Check sheet for the modelled part. Datum: model origin and axes. Units: mm. A direction names the side the tool comes from. Round coordinates to 2 decimals unless told otherwise and drop trailing zeros. Write each loop counter-clockwise with the first axis right and the second up, starting at its lowest first coordinate (ties: lowest second). Pieces come first, ordered by that corner, then holes. Notation, with made-up numbers: (82.25, -34) -> (118.25, -34) arc R15 cw to (118.25, -24) -> close; hole circle Ø1 at (8.5, 70.5). An arc over 180 degrees is marked (long way). One line per item, written item: value.
from build123d import *

# Parameters (mm, degrees)
SKETCH2_R          = 6.746875
CUT_EXTRUDE1_DEPTH = 12.1252


with BuildPart() as part:
    # Sketch1 → Revolve1 (revolve)
    with BuildSketch(Plane.XY):
        with BuildLine():
            Line((0, 0), (0, 11.1252))
            Line((0, 11.1252), (19.05, 11.1252))
            Line((19.05, 11.1252), (19.05, 4.7752))
            Line((19.05, 4.7752), (25.4, 4.7752))
            Line((25.4, 4.7752), (25.4, 0.79375))
            ThreePointArc((25.4, 0.79375), (25.167516008, 0.232483992), (24.60625, 0))
            Line((24.60625, 0), (0, 0))
        make_face()
    revolve(axis=Axis((0, 140.214345547, 0), (0, -1, 0)))

    # Sketch2 → Cut-Extrude1 (cut, through all)
    with BuildSketch(Plane(origin=(0, 11.1252, 0), x_dir=(1, 0, 0), z_dir=(0, 1, 0))):
        Circle(SKETCH2_R)
    extrude(amount=-CUT_EXTRUDE1_DEPTH, mode=Mode.SUBTRACT)


solid = part.part
Item 1: Sectioned sample at B-B on z = 0. Enter the section's corners in (x, y), and give its area (3 significant figures).
Answer:
outline: (-25.4, 0.79) arc R0.79 ccw to (-24.61, 0) -> (-6.75, 0) -> (-6.75, 11.13) -> (-19.05, 11.13) -> (-19.05, 4.78) -> (-25.4, 4.78) -> close; (6.75, 0) -> (24.61, 0) arc R0.79 ccw to (25.4, 0.79) -> (25.4, 4.78) -> (19.05, 4.78) -> (19.05, 11.13) -> (6.75, 11.13) -> close
area: 334 mm^2
Item 2: Sectioned sample at C-C on y = 9.25. Enter the section's corners in (x, z), and give its area (3 significant figures).
Answer:
outline: circle Ø38.1 at (0, 0); hole circle Ø13.49 at (0, 0)
area: 997 mm^2
Item 3: Depth check by flat-ended pin: P1, Ø5, axis at x = 11, y = 4.5, coming from the -Z side; P2, Ø1.5, axis at x = 11, z = -19, coming from the +Y side; P3, Ø4, axis at x = -20, y = 2.5, coming from the +Z side. Enter the tip coordinate at first touch or a pass-through.
Answer:
P1: stops at z = -23.94
P2: stops at y = 4.78
P3: stops at z = 17.92
Item 4: Mould release check, pull along X, two halves, no side actions. Record for faces 3 (the cylindrical face through (-4.97, 5.64, -4.56)), 4 (the flat face through (5, 0, -5)), 5 (the cylindrical face through (-15.12, 7.91, -11.59)): pulls with the +X half, pulls with the -X half, needs draft (parallel to the pull), parting line crosses it, or undercut.
Answer:
face 3: undercut
face 4: needs draft
face 5: parting line crosses it
Item 5: Thickness scan on line 1 (Z direction, x = 0, y = 3); line 2 (Z direction, x = 0, y = 6); line 3 (X direction, y = 8, z = 1). Record the ranges inside material, lowest first.
Answer:
line 1: z = -25.4 to -6.75, 6.75 to 25.4
line 2: z = -19.05 to -6.75, 6.75 to 19.05
line 3: x = -19.02 to -6.67, 6.67 to 19.02
Item 6: Sectioned sample at A-A on x = 0. Enter the section's corners in (y, z).
Answer:
outline: (0, -24.61) arc R0.79 ccw to (0.79, -25.4) -> (4.78, -25.4) -> (4.78, -19.05) -> (11.13, -19.05) -> (11.13, -6.75) -> (0, -6.75) -> close; (0, 6.75) -> (11.13, 6.75) -> (11.13, 19.05) -> (4.78, 19.05) -> (4.78, 25.4) -> (0.79, 25.4) arc R0.79 ccw to (0, 24.61) -> close
Item 7: Tool access check on faces 1 (the flat face through (-4, 4.775, 19)), 2 (the cylindrical face through (-5.506, 2.757, -24.796)). Record the directions out of +Z, -Z, +X, -X, +Y, -Y that give a thin tool (end or side, any length) a straight path to the whole face; none if there is none.
Answer:
face 1: +Y
face 2: +Y, -Y
